The drawing under review shows one solid part. Ordinate dimensions are in mm from its lowest x, y, z. Give positions to 0.01 mm unless a question says otherwise; leave off trailing zeros. Loops run counter-clockwise (first coordinate to the right, second up) from the corner with the lowest first, then second, coordinate; pieces in that order, holes last. Notation, with made-up numbers: M -25.5,-24 L -4.5,-24 A19 cw -4.5,-18 Z; hole C 4.5,64.5 d5. An arc over 180 degrees is marked long. One line per item, written item: value. Start each with the question number.
Q1. We need section D-D on z = 2.2. Write out the cut boundary in (x, y) (3 decimals).
Q2. For pin 1 (0.5 mm diameter, centred on x = 7.5, z = 2, fed in from -Y) (3 decimals); pin 2 (1 mm diameter, centred on x = 9, y = 1.5, fed in from -Z); pin 3 (1.1 mm diameter, centred on x = 7.5, z = 1, fed in from +Y), all flat-tipped, find the tip position at first contact; note any pin that passes through.
Q3. We need section A-A on z = 3.55. Write out the cut boundary in (x, y) (3 decimals), plus the area to 3 significant figures.
Q4. We need section B-B on y = 0.25. Write out the cut boundary in (x, z).
Q5. We need section C-C on x = 7.75. Write out the cut boundary in (y, z) (3 decimals), plus the area to 3 significant figures.
Q6. To check wall thickness, follow line 1 along X through (y, z) = (0.85, 4.35); line 2 along Z through (x, y) = (1.5, 0.9). State the ranges of each line that lie inside material, in increasing order. Write a range as from..to.
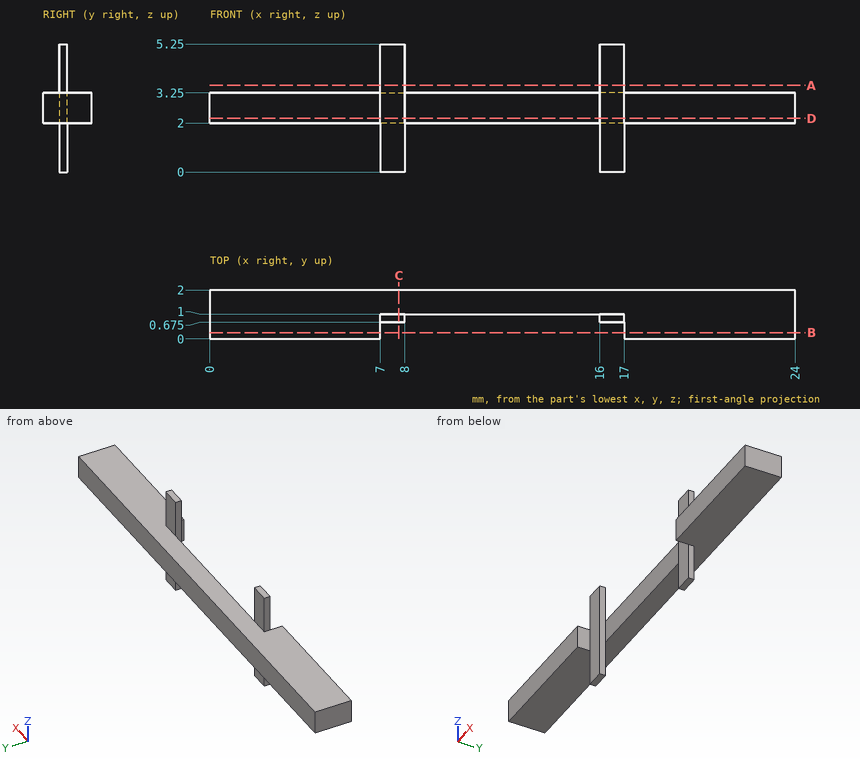
Solved:
1. outline: M 0,0 L 7,0 L 7,0.675 L 8,0.675 L 8,1 L 16,1 L 16,0.675 L 17,0.675 L 17,0 L 24,0 L 24,2 L 0,2 Z
2. pin 1: y = 0.675
2. pin 2: z = 2
2. pin 3: y = 1
3. outline: M 7,0.675 L 8,0.675 L 8,1 L 7,1 Z; M 16,0.675 L 17,0.675 L 17,1 L 16,1 Z
3. area: 0.650 mm2
4. outline: M 0,2 L 7,2 L 7,3.25 L 0,3.25 Z; M 17,2 L 24,2 L 24,3.25 L 17,3.25 Z
5. outline: M 0.675,0 L 1,0 L 1,2 L 2,2 L 2,3.25 L 1,3.25 L 1,5.25 L 0.675,5.25 Z
5. area: 2.96 mm2
6. line 1: 7..8, 16..17
6. line 2: 2..3.25
